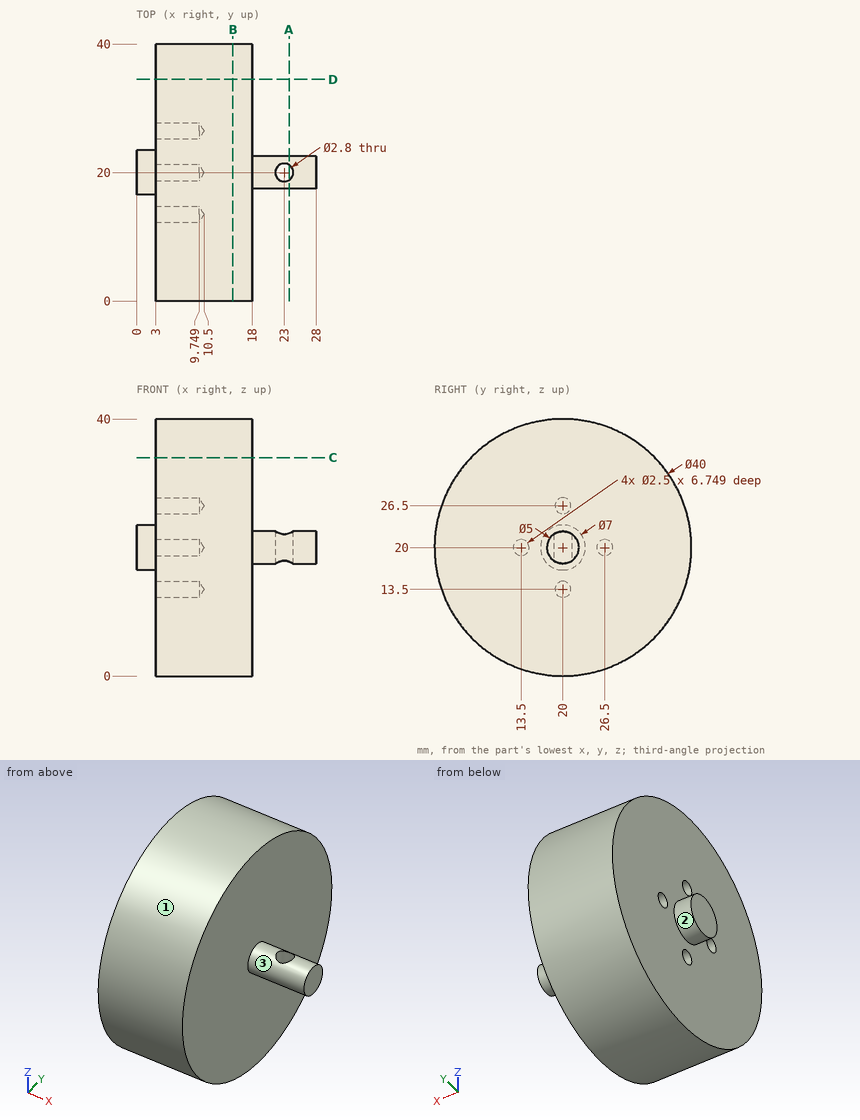
Design review of the part shown in the three views and the two pictorial views. Dimensions are in mm from the part's minimum x, y and z. A direction names the side the tool comes from. Give positions to 0.01 mm unless a question says otherwise; leave off trailing zeros. Loops run counter-clockwise (first coordinate to the right, second up) from the corner with the lowest first, then second, coordinate; pieces in that order, holes last. Notation, with made-up numbers: M 25.25,85.5 L 63.25,85.5 A10 cw 63.25,95.5 Z; hole C 4,-29.75 d4. An arc over 180 degrees is marked long. Put each result on its own line as item: value. Start each with the question number.
(1) Add section C-C, the plane z = 34. Write out the cut boundary in (x, y).
(2) Add section B-B, the plane x = 15. Write out the cut boundary in (y, z).
(3) For pin 1 (2 mm diameter, centred on x = 15.5, z = 9.5, fed in from -Y); pin 2 (4 mm diameter, centred on y = 26.5, z = 20, fed in from -X); pin 3 (6 mm diameter, centred on x = 20.5, z = 9.5, fed in from +Y), all flat-tipped, find the tip position at first contact; note any pin that passes through.
(4) Machinability: for the marked faces 1, 2 and 3, which of the approach directions +Z, -Z, +X, -X, +Y, -Y give a long, thin tool a straight path to every point of the face, cutting with its end or side? Answer none if there is none.
(5) Wall thickness on L1, parallel to Y at x = 6, z = 20; L2, parallel to Y at x = 7.25, z = 26.5; L3, parallel to X at y = 5.5, z = 6.5: over which ranges is each line inside the solid? List them lowest first.
(6) Add section A-A, the plane x = 23.75. Write out the cut boundary in (y, z), then the cut area to 3 significant figures.
(7) Add section D-D, the plane y = 34.5. Write out the cut boundary in (x, z) (3 decimals), then the cut area to 3 significant figures.
Result:
1. outline: M 3,5.72 L 18,5.72 L 18,34.28 L 3,34.28 Z
2. outline: C 20,20 d40
3. pin 1: stops at y = 2.4
3. pin 2: stops at x = 3
3. pin 3: stops at y = 37.94
4. face 1: +X, -X
4. face 2: -X
4. face 3: +X
5. L1: y = 0 to 12.25, 14.75 to 25.25, 27.75 to 40
5. L2: y = 1.09 to 18.75, 21.25 to 38.91
5. L3: x = 3 to 18
6. outline: M 18.82,17.8 L 18.82,22.2 A2.5 ccw Z; M 21.18,17.8 A2.5 ccw 21.18,22.2 Z
6. area: 8.27 mm^2
7. outline: M 3,6.225 L 18,6.225 L 18,33.775 L 3,33.775 Z
7. area: 413 mm^2
